from build123d import *

# Parameters (mm, degrees)
F1_DEPTH = 20
F3_D     = 10
F2_R     = 18
F4_DEPTH = 30
F6_D     = 14
F6_DEPTH = 25
F6_TIP   = 4.2060243332


with BuildPart() as f1:
    # F0 (on Front) → F1 (new body)
    with BuildSketch(Plane.XZ):
        with BuildLine():
            ThreePointArc((-25, 0), (-21.1288563682, 13.3630620956), (-10.7142857143, 22.5876975726))
            Line((-10.7142857143, 22.5876975726), (-39.2857142857, 9.0350790291))
            ThreePointArc((-39.2857142857, 9.0350790291), (-29.6547751618, 8.4515425473), (-25, 0))
        make_face()
        with BuildLine():
            ThreePointArc((39.2857142857, -9.0350790291), (29.6547751618, -8.4515425473), (25, 0))
            ThreePointArc((25, 0), (21.1288563682, -13.3630620956), (10.7142857143, -22.5876975726))
            Line((10.7142857143, -22.5876975726), (39.2857142857, -9.0350790291))
        make_face()
        with BuildLine():
            Line((-39.2857142857, -9.0350790291), (-10.7142857143, -22.5876975726))
            ThreePointArc((-10.7142857143, -22.5876975726), (-21.1288563682, -13.3630620956), (-25, 0))
            ThreePointArc((-25, 0), (-29.6547751618, -8.4515425473), (-39.2857142857, -9.0350790291))
        make_face()
        with BuildLine():
            ThreePointArc((10.7142857143, -22.5876975726), (21.1288563682, -13.3630620956), (25, 0))
            ThreePointArc((25, 0), (21.1288563682, 13.3630620956), (10.7142857143, 22.5876975726))
            ThreePointArc((10.7142857143, 22.5876975726), (0, 25), (-10.7142857143, 22.5876975726))
            ThreePointArc((-10.7142857143, 22.5876975726), (-21.1288563682, 13.3630620956), (-25, 0))
            ThreePointArc((-25, 0), (-21.1288563682, -13.3630620956), (-10.7142857143, -22.5876975726))
            ThreePointArc((-10.7142857143, -22.5876975726), (0, -25), (10.7142857143, -22.5876975726))
        make_face()
        with BuildLine():
            ThreePointArc((-39.2857142857, -9.0350790291), (-29.6547751618, -8.4515425473), (-25, 0))
            ThreePointArc((-25, 0), (-29.6547751618, 8.4515425473), (-39.2857142857, 9.0350790291))
            ThreePointArc((-39.2857142857, 9.0350790291), (-45, 0), (-39.2857142857, -9.0350790291))
        make_face()
        with BuildLine():
            ThreePointArc((39.2857142857, 9.0350790291), (29.6547751618, 8.4515425473), (25, 0))
            ThreePointArc((25, 0), (29.6547751618, -8.4515425473), (39.2857142857, -9.0350790291))
            ThreePointArc((39.2857142857, -9.0350790291), (43.4515425473, -5.3452248382), (45, 0))
            ThreePointArc((45, 0), (43.4515425473, 5.3452248382), (39.2857142857, 9.0350790291))
        make_face()
        with BuildLine():
            ThreePointArc((10.7142857143, 22.5876975726), (21.1288563682, 13.3630620956), (25, 0))
            ThreePointArc((25, 0), (29.6547751618, 8.4515425473), (39.2857142857, 9.0350790291))
            Line((39.2857142857, 9.0350790291), (10.7142857143, 22.5876975726))
        make_face()
    extrude(amount=F1_DEPTH)

    # F3 (through all)
    with Locations(Plane.XZ.offset(20)):
        with Locations((-35, 0), (35, 0)):
            Hole(F3_D / 2)

    # F2 (on face) → F4 (join)
    with BuildSketch(Plane.XZ.offset(20)):
        Circle(F2_R)
    extrude(amount=F4_DEPTH)

    # F6
    with Locations(Plane.XZ.offset(50)):
        with Locations((0, 0)):
            Hole(F6_D / 2, depth=F6_DEPTH)
            with Locations((0, 0, -(F6_DEPTH + F6_TIP / 2))):  # 118° drill point
                Cone(0, F6_D / 2, F6_TIP, mode=Mode.SUBTRACT)


solid = f1.part
Can you work these out from the model? Positions are in its coordinate system, mm. A direction names the side the tool comes from. Coordinates: 2 decimals unless noted, no trailing zeros. Loops run counter-clockwise (first coordinate to the right, second up) from the corner with the lowest first, then second, coordinate; pieces in that order, holes last. Notation, with made-up numbers: (74.25, 32) - (78.25, 32) arc R12 cw to (78.25, 36) - close; hole circle Ø5 at (29.25, 55). An arc over 180 degrees is marked (long way). Answer as a JSON object with one key per item and string values. Group by question number.
Item 1: If we section it at A-A (y = -13.5): List the corners of the cut face in (x, z) for me, plus the area to 3 significant figures.
Item 2: If we section it at D-D (z = 16.5): List the corners of the cut face in (x, y) for me.
Item 3: If we section it at C-C (y = -46): List the corners of the cut face in (x, z) for me.
Item 4: For pin 1 (12.5 mm diameter, centred on x = 0, z = 0, fed in from -Y); pin 2 (8 mm diameter, centred on x = 24.5, z = 20, fed in from -Y); pin 3 (12 mm diameter, centred on x = 6.5, z = -15.5, fed in from +Y); pin 4 (4 mm diameter, centred on y = -28, z = -4, fed in from +X), each with a flat end and sliding along its axis, tell me the tip position at first contact or that it passes through.
Item 5: If we mould it in two halves opening along Z, with no side actions, what happens to faces 3 (the face through (40, -10, 0)), 4 (the face through (-1, 0, 0)), 5 (the face through (-0.264, -21.524, -1.187)), 6 (the face through (25.2, -9.86, 15.717))? For each: released by +Z, released by -Z, zero draft, split by the parting line, or undercut.
Item 6: If we section it at B-B (x = -32): List the corners of the cut face in (y, z) for me, plus the area to 3 significant figures.
Item 7: If I drill on L1, parallel to Z at x = 0, y = -30; L2, parallel to X at y = -12, z = 3.5; L3, parallel to X at y = -19, z = 2.5, over which ranges is the centre line in solid material (lowest first)? Write a range as from..to.
Item 8: On a 3-axis mill with a long thin cutter (end or side, diameter ignored), from which of +Z, -Z, +X, -X, +Y, -Y can I reach the whole of each face in a straight line? I mean faces 1 (the face through (0, -10, 25)), 2 (the face through (-11, -20, 17)). Say none if no direction works.
Returned:
{
 "1": {"outline": "(-39.29, -9.04) - (-10.71, -22.59) arc R25 ccw to (10.71, -22.59) - (39.29, -9.04) arc R10 ccw to (39.29, 9.04) - (10.71, 22.59) arc R25 ccw to (-10.71, 22.59) - (-39.29, 9.04) arc R10 ccw to start; hole circle Ø10 at (-35, 0); hole circle Ø10 at (35, 0)", "area": "2,840 mm²"},
 "2": {"outline": "(-23.55, -20) - (-7.19, -20) - (-7.19, -50) - (7.19, -50) - (7.19, -20) - (23.55, -20) - (23.55, 0) - (-23.55, 0) - close"},
 "3": {"outline": "circle Ø36 at (0, 0); hole circle Ø14 at (0, 0)"},
 "4": {"pin 1": "stops at y = -24.55", "pin 2": "stops at y = -20", "pin 3": "stops at y = 0", "pin 4": "stops at x = 17.89"},
 "5": {"face 3": "undercut", "face 4": "zero draft", "face 5": "undercut", "face 6": "released by +Z"},
 "6": {"outline": "(-20, -12.49) - (0, -12.49) - (0, -4) - (-20, -4) - close; (-20, 4) - (0, 4) - (0, 12.49) - (-20, 12.49) - close", "area": "340 mm²"},
 "7": {"L1": "z = -18..-7, 7..18", "L2": "x = -44.37..-38.57, -31.43..31.43, 38.57..44.37", "L3": "x = -44.68..-39.33, -30.67..30.67, 39.33..44.68"},
 "8": {"face 1": "+Z, +Y, -Y", "face 2": "-Y"}
}
